from build123d import *

# Parameters (mm, degrees)
SKETCH_R        = 1.6
PAD_DEPTH       = 20
PAD001_DEPTH    = 45
SKETCH002_R     = 4.075
POCKET_DEPTH    = 31.803267
POCKET001_DEPTH = 20.001
SKETCH004_R     = 1.6
POCKET002_DEPTH = 21.561
FILLET_R        = 3
POCKET003_DEPTH = 3.2
POCKET004_DEPTH = 3.2


with BuildPart() as part:
    # Sketch → Pad (new body)
    with BuildSketch(Plane.XY):
        Polygon((22.5, 10), (22.5, -10), (-22.5, -10), (-22.5, 10), (-8.552884, 10), (-1.023266, 13.11887), (0.268613, 10), align=None)
        with Locations((-2.487442, 6.005217)):
            Circle(SKETCH_R, mode=Mode.SUBTRACT)
        with Locations((2.487442, -6.005217)):
            Circle(SKETCH_R, mode=Mode.SUBTRACT)
    extrude(amount=PAD_DEPTH)

    # Sketch001 (on Face3 of Pad) → Pad001 (join)
    with BuildSketch(Plane(origin=(-22.5, 0, 0), x_dir=(0, -1, 0), z_dir=(-1, 0, 0))):
        Polygon((10, 10), (10, 14.74), (11.56, 12.94), (11.56, 7.06), (10, 5.26), align=None)
    extrude(amount=-PAD001_DEPTH)

    # Sketch002 (on Face14 of Pad001) → Pocket (cut, through all)
    with BuildSketch(Plane(origin=(-4.788075, 11.559435, 0), x_dir=(-0.92388, -0.382683, 0), z_dir=(-0.382683, 0.92388, 0))):
        with Locations((0, 10)):
            Circle(SKETCH002_R)
    extrude(amount=-POCKET_DEPTH, mode=Mode.SUBTRACT)

    # Sketch003 (on Face6 of Pocket) → Pocket001 (cut, through all)
    with BuildSketch(Plane(origin=(0, 0, 0), x_dir=(1, 0, 0), z_dir=(0, 0, -1))):
        Polygon((-8.552884, -10), (-1.023266, -13.11887), (0.268613, -10), align=None)
    extrude(amount=-POCKET001_DEPTH, mode=Mode.SUBTRACT)

    # Sketch004 (on Face2 of Pocket001) → Pocket002 (cut, through all)
    with BuildSketch(Plane(origin=(0, 10, 0), x_dir=(-1, 0, 0), z_dir=(0, 1, 0))):
        with Locations((-17.186, 10)):
            Circle(SKETCH004_R)
        with Locations((17.186, 10)):
            Circle(SKETCH004_R)
    extrude(amount=-POCKET002_DEPTH, mode=Mode.SUBTRACT)

    # Fillet
    fillet_edges = [part.edges().sort_by_distance(p)[0] for p in [
        (-22.5, 10, 10),
        (22.5, 10, 10),
    ]]
    fillet(fillet_edges, radius=FILLET_R)

    # Sketch005 (on Face2 of Fillet) → Pocket003 (cut)
    with BuildSketch(Plane(origin=(0, 0, 0), x_dir=(1, 0, 0), z_dir=(0, 0, -1))):
        Polygon((5.720604, 6.005217), (4.104023, 8.805217), (0.870862, 8.805217), (-0.745719, 6.005217), (0.870862, 3.205217), (4.104023, 3.205217), align=None)
        Polygon((-5.720604, -6.005217), (-4.104023, -8.805217), (-0.870862, -8.805217), (0.745719, -6.005217), (-0.870862, -3.205217), (-4.104023, -3.205217), align=None)
    extrude(amount=-POCKET003_DEPTH, mode=Mode.SUBTRACT)

    # Sketch006 (on Face5 of Pocket003) → Pocket004 (cut)
    with BuildSketch(Plane.XY.offset(20)):
        Polygon((0.745719, 6.005217), (-0.870862, 8.805217), (-4.104023, 8.805217), (-5.720604, 6.005217), (-4.104023, 3.205217), (-0.870862, 3.205217), align=None)
        Polygon((5.720604, -6.005217), (4.104023, -3.205217), (0.870862, -3.205217), (-0.745719, -6.005217), (0.870862, -8.805217), (4.104023, -8.805217), align=None)
    extrude(amount=-POCKET004_DEPTH, mode=Mode.SUBTRACT)


solid = part.part
Verification items for the finished model (mm, model axes). A direction names the side the tool comes from. Coordinates: 2 decimals unless noted, no trailing zeros. Order: outer loops, then holes, each group sorted by start corner. A loop starts at its lowest first (then second) coordinate and runs counter-clockwise, first axis right, second up.
Item 1: Release check for a two-part mould opening along Y. For faces 1 (the face through (0, -10, 3)), 2 (the face through (-3.211, -2.085, 8.439)), 3 (the face through (0, 10, 8)), 4 (the face through (22.5, -2, 10)) record: +Y half, -Y half, draft (parallel to the pull), parting line (faces both ways), or undercut.
Filled in:
face 1: -Y half
face 2: undercut
face 3: +Y half
face 4: draft
Item 2: Section check A-A, the plane z = 16.25. Enter the section's corners in (x, y).
Filled in:
outline: (-22.5, -10) - (22.5, -10) - (22.5, 7) arc R3 ccw to (19.5, 10) - (-19.5, 10) arc R3 ccw to (-22.5, 7) - close; hole circle Ø3.2 at (-2.49, 6.01); hole circle Ø3.2 at (2.49, -6.01)
Item 3: Section check B-B, the plane x = -9. Enter the section's corners in (y, z).
Filled in:
outline: (-11.56, 7.06) - (-10, 5.26) - (-10, 0) - (10, 0) - (10, 20) - (-10, 20) - (-10, 14.74) - (-11.56, 12.94) - close
Item 4: Depth check by flat-ended pin: pin 1 (4 mm diameter, centred on x = 2.49, y = -6.01, fed in from +Z); pin 2 (5 mm diameter, centred on x = 17.186, z = 10, fed in from +Y); pin 3 (1 mm diameter, centred on x = 2, z = 1.5, fed in from -Y); pin 4 (1.7 mm diameter, centred on x = 4, y = -6.5, fed in from -Z). Enter the tip coordinate at first touch or a pass-through.
Filled in:
pin 1: stops at z = 16.8
pin 2: stops at y = 10
pin 3: stops at y = -10
pin 4: stops at z = 3.2
Item 5: Section check C-C, the plane x = -17. Enter the section's corners in (y, z).
Filled in:
outline: (-11.56, 7.06) - (-10, 5.26) - (-10, 0) - (10, 0) - (10, 8.41) - (-11.56, 8.41) - close; (-11.56, 11.59) - (10, 11.59) - (10, 20) - (-10, 20) - (-10, 14.74) - (-11.56, 12.94) - close
Item 6: Access from +Z, -Z, +X, -X, +Y, -Y to the whole of each face (thin tool, end or side, straight path). Record for faces 5 (the face through (-4.901, 7.425, 18.422)), 6 (the face through (4.01, -5.52, 4.7)), 7 (the face through (0.07, -7.42, 1.58)).
Filled in:
face 5: +Z
face 6: +Z, -Z
face 7: -Z
Item 7: Section check D-D, the plane z = 12.5. Enter the section's corners in (x, y), then the cut area to 3 significant figures.
Filled in:
outline: (-22.5, -11.56) - (1.31, -11.56) - (-7.63, 10) - (-19.5, 10) arc R3 ccw to (-22.5, 7) - close; (-0.66, 10) - (8.27, -11.56) - (22.5, -11.56) - (22.5, 7) arc R3 ccw to (19.5, 10) - close
area: 816 mm2
Item 8: Material ranges on L1, parallel to Y at x = 4, z = 2.5; L2, parallel to X at y = -1.5, z = 9.25; L3, parallel to X at y = -3.5, z = 10.75, recorded low to high.
Filled in:
L1: y = -10 to -8.81, -3.21 to 10
L2: x = -22.5 to -18.6, -15.77 to -3.71, 4.96 to 15.77, 18.6 to 22.5
L3: x = -22.5 to -18.6, -15.77 to -2.89, 5.79 to 15.77, 18.6 to 22.5
